Design review of the part built by this model. Coordinates are the model's own, in mm. Face numbers are marked on the shaded views. A direction names the side the tool comes from. Coordinates: 2 decimals unless noted, no trailing zeros. Write each loop counter-clockwise with the first axis right and the second up, starting at its lowest first coordinate (ties: lowest second). Pieces come first, ordered by that corner, then holes.
Q1. Add section C-C, the plane z = -5. Give the boundary of the cut face in (x, y).
Q2. Add section A-A, the plane x = -5. Give the boundary of the cut face in (y, z), plus the area to 3 significant figures.
Q3. To check wall thickness, follow probe 1 along X at (y, z) = (1.5, -5); probe 2 along Z at (x, y) = (-5, 1.5); probe 3 along X at (y, z) = (1.3, -8). State the ranges of each line that lie inside material, in increasing order.
Q4. Machinability: for the marked faces 1, 2 and 3, which of the approach directions +Z, -Z, +X, -X, +Y, -Y give a long, thin tool a straight path to every point of the face, cutting with its end or side? Answer none if there is none.
Q5. The part is to be moulded in two halves that separate along Z. For the marked faces 4, 5 and 6, say which applies: +Z half, -Z half, draft (parallel to the pull), parting line (faces both ways), or undercut.
Q6. Clearance check with a flat-ended pin moving along its axis: pin 1 Ø1.5 at (y, z) = (1.5, -7) entering from +X. State where the tip first meets the part, or that it passes through.
Q7. Add section B-B, the plane y = 2.05. Give the boundary of the cut face in (x, z).
Q8. Add section D-D, the plane z = -24. Give the boundary of the cut face in (x, y).
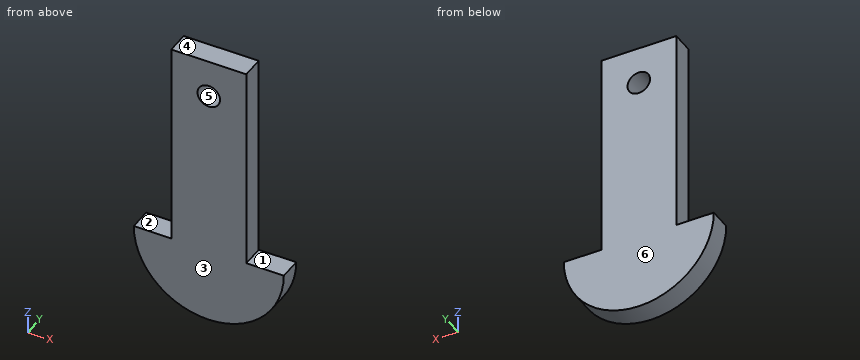
Autodesk Inventor part; units mm, degrees
ref_plane "YZ Plane" through (0, 0, 0) normal (1, 0, 0) x (0, 1, 0)
ref_plane "XZ Plane" through (0, 0, 0) normal (0, 1, 0) x (-1, 0, 0)
ref_plane "XY Plane" through (0, 0, 0) normal (0, 0, 1) x (1, 0, 0)
sketch "Sketch1" plane through (0, 0, 0) normal (0, 1, 0) x (-1, 0, 0)
  line L0 (0, 0) -> (10, 0)
  line L1 (10, 0) -> (10, -27.5)
  line L2 (10, -27.5) -> (0, -27.5)
  line L3 (0, -27.5) -> (0, 0)
  line L4 (10, -27.5) -> (15, -27.5)
  line L5 (0, -27.5) -> (-5, -27.5)
  arc A0 (-5, -27.5) -> (15, -27.5) centre (5, -27.5143) ccw
  dimension "d0" = 10
  dimension "d1" = 27.5
  dimension "d2" = 5
  dimension "d3" = 5
extrude "Extrusion1" add sketch "Sketch1" along normal blind 3
sketch "Sketch2" plane through (0, 3, 0) normal (0, 1, 0) x (1, 0, 0)
  circle A0 centre (-5, 5) radius 1.5
  line L0 (-10, 0) -> (0, 0)
  line L1 (-10, 27.5) -> (-10, 0)
  dimension "d6" = 3
  dimension "d7" = 5
  dimension "d8" = 5
hole "Hole1" at (-5, 3, -5) direction (0, -1, 0) diameter 3 end through all
properties part number "fixing"
Here are the results:
1. outline: (-10, 0) - (-6.5, 0) - (-6.5, 3) - (-10, 3) - close; (-3.5, 0) - (0, 0) - (0, 3) - (-3.5, 3) - close
2. outline: (0, -37.51) - (3, -37.51) - (3, -6.5) - (0, -6.5) - close; (0, -3.5) - (3, -3.5) - (3, 0) - (0, 0) - close
2. area: 104 mm2
3. probe 1: x = -10 to -6.5, -3.5 to 0
3. probe 2: z = -37.51 to -6.5, -3.5 to 0
3. probe 3: x = -10 to 0
4. face 1: +Z, +X, +Y, -Y
4. face 2: +Z, -X, +Y, -Y
4. face 3: +Z, -Z, +X, -X, -Y
5. face 4: +Z half
5. face 5: undercut
5. face 6: draft
6. pin 1: stops at x = 0
7. outline: (-15, -27.5) arc R10 ccw to (5, -27.5) - (0, -27.5) - (0, 0) - (-10, 0) - (-10, -27.5) - close; hole circle Ø3 at (-5, -5)
8. outline: (-10, 0) - (0, 0) - (0, 3) - (-10, 3) - close
